```python
from build123d import *

# Parameters (mm, degrees)
EXTRUDE_1_DEPTH      = 4
EXTRUDE_1_DEPTH_BACK = 4
SKETCH_1_R           = 0.75
SKETCH_2_R           = 2
EXTRUDE_2_DEPTH      = 1
EXTRUDE_START        = 1
SKETCH_3_R           = 2
EXTRUDE_3_DEPTH      = 1
SKETCH_6_W           = 1.5
SKETCH_6_H           = 3
EXTRUDE_6_DEPTH      = 1
SKETCH_7_W           = 1.5
SKETCH_7_H           = 3
EXTRUDE_8_DEPTH      = 1
SKETCH_8_W           = 3
SKETCH_8_H           = 2
EXTRUDE_9_DEPTH      = 0.5
EXTRUDE_10_DEPTH     = 1
EXTRUDE_START_2      = 7
EXTRUDE_11_DEPTH     = 1
CUT_EXTRUDE_1_DEPTH  = 12.338430226
EXTRUDE_12_DEPTH     = 1


with BuildPart() as part:
    # 草图1 → 凸台-拉伸1 (new, two sides: drawn at the far end of the back side and taken through both)
    with BuildSketch(Plane(origin=(0, 0, 0), x_dir=(1, 0, 0), z_dir=(0, 1, 0)).offset(-EXTRUDE_1_DEPTH_BACK)):
        with Locations(Location((0, 0, 0), (0, 0, 270))):
            Circle(SKETCH_1_R)
    extrude(amount=EXTRUDE_1_DEPTH + EXTRUDE_1_DEPTH_BACK)

    # 草图2 → 凸台-拉伸2 (add)
    with BuildSketch(Plane(origin=(0, 4, 0), x_dir=(-1, 0, 0), z_dir=(0, 1, 0))):
        with Locations(Location((0, 0, 0), (0, 0, 90))):
            Circle(SKETCH_2_R)
    extrude(amount=EXTRUDE_2_DEPTH)

    # 草图3 → 凸台-拉伸3 (add)
    with BuildSketch(Plane.XZ.offset(4).offset(EXTRUDE_START)):
        with Locations(Location((0, 0, 0), (0, 0, 90))):
            Circle(SKETCH_3_R)
    extrude(amount=-EXTRUDE_3_DEPTH)

    # 草图6 → 凸台-拉伸6 (add)
    with BuildSketch(Plane(origin=(0, 5, 0), x_dir=(-1, 0, 0), z_dir=(0, 1, 0))):
        with Locations((1.75, 0)):
            Rectangle(SKETCH_6_W, SKETCH_6_H)
    extrude(amount=-EXTRUDE_6_DEPTH)

    # 草图7 → 凸台-拉伸8 (add)
    with BuildSketch(Plane.XZ.offset(5)):
        with Locations((-1.75, 0)):
            Rectangle(SKETCH_7_W, SKETCH_7_H)
    extrude(amount=-EXTRUDE_8_DEPTH)

    # 草图8 → 凸台-拉伸9 (add)
    with BuildSketch(Plane.ZY.offset(2.5)):
        with Locations((0, 4)):
            Rectangle(SKETCH_8_W, SKETCH_8_H)
        with Locations((0, -4)):
            Rectangle(SKETCH_8_W, SKETCH_8_H)
    extrude(amount=-EXTRUDE_9_DEPTH)

    # 草图9 → 凸台-拉伸10 (add)
    with BuildSketch(Plane.XZ.offset(-3)):
        with BuildLine():
            Line((-2.5, -1.5), (-3.277124344, -1.5))
            ThreePointArc((-3.277124344, -1.5), (-6.6, 0), (-3.277124344, 1.5))
            Line((-3.277124344, 1.5), (-2.5, 1.5))
            Line((-2.5, 1.5), (-2.5, -1.5))
        make_face()
    extrude(amount=-EXTRUDE_10_DEPTH)

    # 草图9<2> → 凸台-拉伸11 (add)
    with BuildSketch(Plane.XZ.offset(-3).offset(EXTRUDE_START_2)):
        with BuildLine():
            Line((-2.5, -1.5), (-3.277124344, -1.5))
            ThreePointArc((-3.277124344, -1.5), (-6.6, 0), (-3.277124344, 1.5))
            Line((-3.277124344, 1.5), (-2.5, 1.5))
            Line((-2.5, 1.5), (-2.5, -1.5))
        make_face()
    extrude(amount=-EXTRUDE_11_DEPTH)

    # 草图10 → 切除-拉伸1 (cut, through all)
    with BuildSketch(Plane(origin=(0, 4, 0), x_dir=(-1, 0, 0), z_dir=(0, 1, 0))):
        with BuildLine():
            Line((5.35, 0), (5.35, -1.854049622))
            ThreePointArc((5.35, -1.854049622), (4.548070298, -1.999325713), (3.754763477, -1.812615574))
            Line((3.754763477, -1.812615574), (4.283036304, -0.67973084))
            ThreePointArc((4.283036304, -0.67973084), (4.197025294, 0.632543584), (5.35, 0))
        make_face()
    extrude(amount=-CUT_EXTRUDE_1_DEPTH, mode=Mode.SUBTRACT)

    # 草图11 → 凸台-拉伸12 (add)
    with BuildSketch(Plane(origin=(0, 5, 0), x_dir=(1, 0, 0), z_dir=(0, 1, 0))):
        with BuildLine():
            Line((-2, 0), (2, 0))
            Line((2, 0), (2, 2))
            Line((2, 2), (1.5, 2))
            Line((1.5, 2), (1.5, 2.677124344))
            ThreePointArc((1.5, 2.677124344), (1.780042303, 3.088161527), (1.95, 3.555590279))
            Line((1.95, 3.555590279), (1.95, 4.5))
            Line((1.95, 4.5), (-1.95, 4.5))
            Line((-1.95, 4.5), (-1.95, 3.555590279))
            ThreePointArc((-1.95, 3.555590279), (-1.780042303, 3.088161527), (-1.5, 2.677124344))
            Line((-1.5, 2.677124344), (-1.5, 2))
            Line((-1.5, 2), (-2, 2))
            Line((-2, 2), (-2, 0))
        make_face()
    extrude_12 = extrude(amount=-EXTRUDE_12_DEPTH)

    # 镜向1: 凸台-拉伸12 across plane
    add(extrude_12.mirror(Plane.ZX))


solid = part.part
```
Build history of the part. All positions in model axes, mm. A direction names the side the tool comes from. Round coordinates to 2 decimals unless told otherwise and drop trailing zeros. Loops run counter-clockwise (first coordinate to the right, second up) from the corner with the lowest first, then second, coordinate; pieces in that order, holes last.
Item 1: Saw through at C-C (x = 0). List the corners of the cut face in (y, z).
Item 2: Two-plate mould, pull along X, no slides. Class faces 6 (the face through (0, -4.5, -4.5)), 7 (the face through (-5.35, 3.5, -0.9)), 8 (the face through (-1.78, -4.51, -3.09)): released by +X, released by -X, zero draft, split by the parting line, or undercut.
Item 3: Saw through at A-A (x = -4.6). List the corners of the cut face in (y, z).
Item 4: Drill centre lines: line 1 along X through (y, z) = (-3.65, 0); line 2 along Y through (x, z) = (-1, -3.5); line 3 along Y through (x, z) = (-5.5, -1.25). Where is each one in solid material? Low to high.
Item 5: Saw through at D-D (z = 0.5). List the corners of the cut face in (x, y).
Item 6: Saw through at B-B (z = -4). List the corners of the cut face in (x, y).
Item 7: Pin check, flat tips, straight feed: P1, Ø3, axis at x = -3, y = 3.5, coming from the +Z side; P2, Ø1.6, axis at x = -2, y = -4, coming from the +Z side; P3, Ø1, axis at y = -4.5, z = -4, coming from the +X side; P4, Ø5, axis at x = -1.5, y = -3.5, coming from the -Z side. Stop position of each tip, or through.
Item 8: Which spindle directions (+Z, -Z, +X, -X, +Y, -Y) get a long thin tool onto all of the face, cutting with end or side? Do faces 1 (the face through (-2.3, -4, 1.5)), 2 (the face through (-2.5, -4.5, 0)), 3 (the face through (1.95, -4.5, -4)), 4 (the face through (-4, -3, 1)), 5 (the face through (-2.5, 3.8, -1.5)). Say none if no direction does.
Worked answers:
1. outline: (-5, -4.5) - (-4, -4.5) - (-4, -0.75) - (4, -0.75) - (4, -4.5) - (5, -4.5) - (5, 2) - (4, 2) - (4, 0.75) - (-4, 0.75) - (-4, 2) - (-5, 2) - close
2. face 6: zero draft
2. face 7: undercut
2. face 8: released by -X
3. outline: (-4, 0.75) - (-3, 0.75) - (-3, 2) - (-4, 2) - close; (3, 0.75) - (4, 0.75) - (4, 2) - (3, 2) - close
4. line 1: x = -6.6 to -5.35, -3.85 to -2, -0.75 to 0.75
4. line 2: y = -5 to -4, 4 to 5
4. line 3: y = -4 to -3, 3 to 4
5. outline: (-6.54, -4) - (-5.16, -4) - (-5.16, -3) - (-6.54, -3) - close; (-6.54, 3) - (-5.16, 3) - (-5.16, 4) - (-6.54, 4) - close; (-4.04, -4) - (-2.5, -4) - (-2.5, -5) - (1.94, -5) - (1.94, -4) - (0.56, -4) - (0.56, 4) - (1.94, 4) - (1.94, 5) - (-2.5, 5) - (-2.5, 4) - (-4.04, 4) - (-4.04, 3) - (-2, 3) - (-2, 4) - (-0.56, 4) - (-0.56, -4) - (-2, -4) - (-2, -3) - (-4.04, -3) - close
6. outline: (-1.95, -5) - (1.95, -5) - (1.95, -4) - (-1.95, -4) - close; (-1.95, 4) - (1.95, 4) - (1.95, 5) - (-1.95, 5) - close
7. P1: stops at z = 2
7. P2: stops at z = 1.6
7. P3: stops at x = 1.95
7. P4: stops at z = -4.5
8. face 1: +Z, +Y, -Y
8. face 2: +Z, -Z, -X, -Y
8. face 3: -Z, +X, +Y, -Y
8. face 4: +Z, -Z, -X
8. face 5: -Z, +Y, -Y
